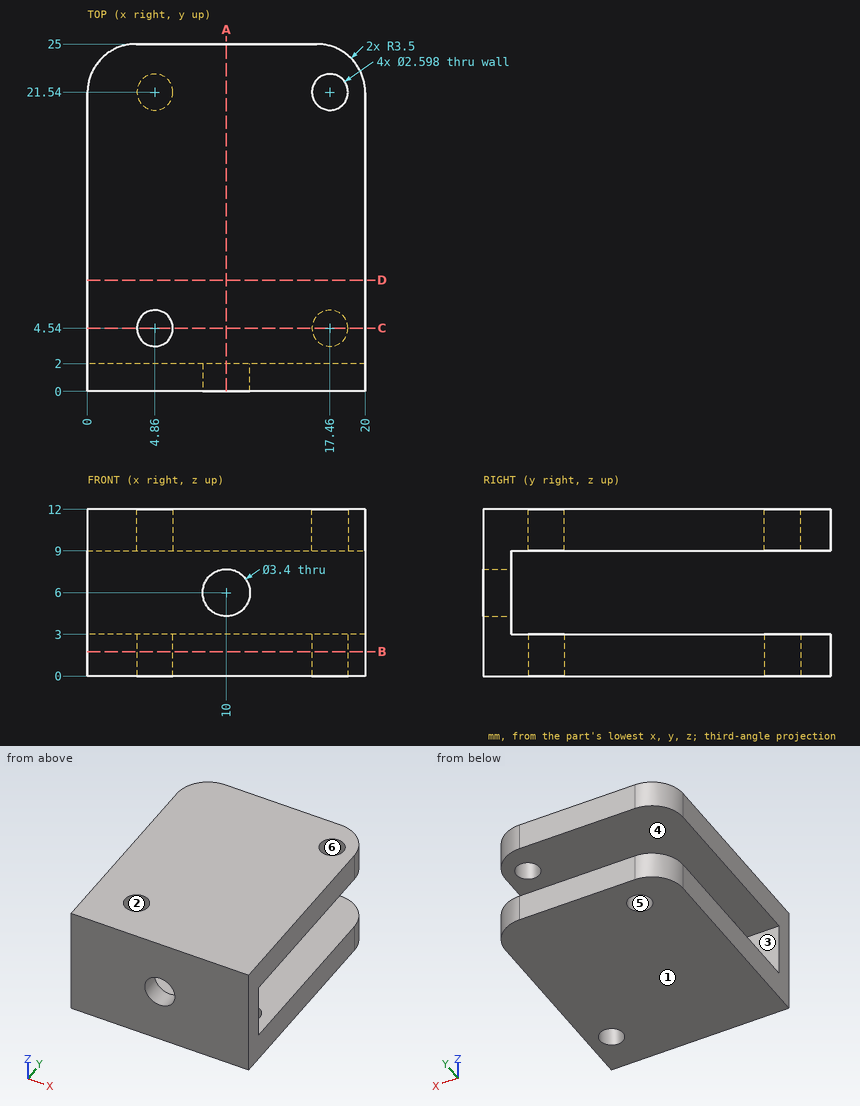
Source: three-view drawing plus pictorial views. Frame: mm from the lowest corner of the part. A direction names the side the tool comes from. Give positions to 0.01 mm unless a question says otherwise; leave off trailing zeros. Order: outer loops, then holes, each group sorted by start corner. A loop starts at its lowest first (then second) coordinate and runs counter-clockwise, first axis right, second up.
1. Mould query, pull axis Z, two halves, no side actions, for the marked faces 1, 2 and 3. Classes: released by +Z, released by -Z, zero draft, split by the parting line, or undercut.
Derived:
face 1: released by -Z
face 2: zero draft
face 3: undercut
2. Section A-A on x = 10. Return the cut outline in (y, z).
Derived:
outline: (0, 0) - (25, 0) - (25, 3) - (2, 3) - (2, 4.3) - (0, 4.3) - close; (0, 7.7) - (2, 7.7) - (2, 9) - (25, 9) - (25, 12) - (0, 12) - close
3. Reachability of the marked faces 4, 5 and 6 from +Z, -Z, +X, -X, +Y, -Y: full face, straight path, thin tool, end or side. Return the list, or none.
Derived:
face 4: +X, -X, +Y
face 5: -Z
face 6: +Z
4. Section B-B on z = 1.75. Return the cut outline in (x, y).
Derived:
outline: (0, 0) - (20, 0) - (20, 21.5) arc R3.5 ccw to (16.5, 25) - (3.5, 25) arc R3.5 ccw to (0, 21.5) - close; hole circle Ø2.6 at (4.86, 21.54); hole circle Ø2.6 at (17.46, 4.54)
5. Material intervals for L1, parallel to Y at x = 4.86, z = 9.8; L2, parallel to Z at x = 14.5, y = 14.25; L3, parallel to Z at x = 10, y = 0.6, sorted ascending.
Derived:
L1: y = 0 to 3.24, 5.84 to 25
L2: z = 0 to 3, 9 to 12
L3: z = 0 to 4.3, 7.7 to 12
6. Section C-C on y = 4.54. Return the cut outline in (x, z).
Derived:
outline: (0, 0) - (16.16, 0) - (16.16, 3) - (0, 3) - close; (0, 9) - (3.56, 9) - (3.56, 12) - (0, 12) - close; (6.16, 9) - (20, 9) - (20, 12) - (6.16, 12) - close; (18.76, 0) - (20, 0) - (20, 3) - (18.76, 3) - close
7. Section D-D on y = 8. Return the cut outline in (x, z), and give its area (3 significant figures).
Derived:
outline: (0, 0) - (20, 0) - (20, 3) - (0, 3) - close; (0, 9) - (20, 9) - (20, 12) - (0, 12) - close
area: 120 mm2
